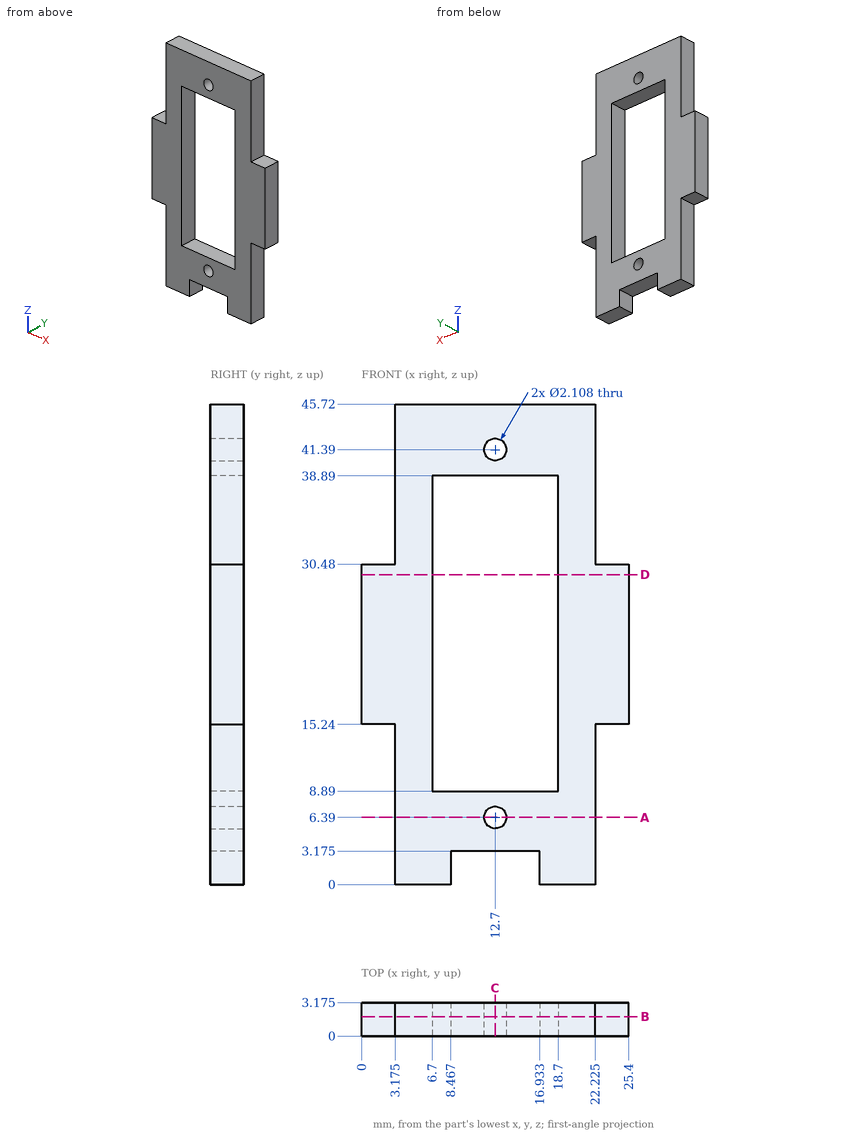
Design review of the part shown in the three views and the two pictorial views. Dimensions are in mm from the part's minimum x, y and z. Coordinates: 2 decimals unless noted, no trailing zeros. Write each loop counter-clockwise with the first axis right and the second up, starting at its lowest first coordinate (ties: lowest second). Pieces come first, ordered by that corner, then holes. Notation, with made-up numbers: (-7.5, 34.5) -> (14.5, 34.5) arc R26 ccw to (14.5, 68.5) -> close; hole circle Ø7 at (-5.5, 13). An arc over 180 degrees is marked (long way). Answer in a Markdown table with one row per item.
1. Clearance check with flat-ended pins moving along their axes: pin 1 Ø1 at (y, z) = (1, 10) entering from +X (3 decimals); pin 2 Ø1.6 at (x, y) = (13, 1) entering from -Z (3 decimals); pin 3 Ø1.6 at (y, z) = (1, 6.5) entering from -X (3 decimals); pin 4 Ø1 at (y, z) = (2, 30) entering from -X. State where each tip first meets the part, or that it passes through.
Answers below:
| item | result |
|---|---|
| pin 1 | stops at x = 22.225 |
| pin 2 | stops at z = 3.175 |
| pin 3 | stops at x = 3.175 |
| pin 4 | stops at x = 0 |
2. We need section D-D, the plane z = 29.5. State the section outline as (x, y) points (1 decimal).
Answers below:
| item | result |
|---|---|
| outline | (0, 0) -> (6.7, 0) -> (6.7, 3.2) -> (0, 3.2) -> close; (18.7, 0) -> (25.4, 0) -> (25.4, 3.2) -> (18.7, 3.2) -> close |
3. We need section C-C, the plane x = 12.7. State the section outline as (y, z) points (1 decimal).
Answers below:
| item | result |
|---|---|
| outline | (0, 3.2) -> (3.2, 3.2) -> (3.2, 5.3) -> (0, 5.3) -> close; (0, 7.4) -> (3.2, 7.4) -> (3.2, 8.9) -> (0, 8.9) -> close; (0, 38.9) -> (3.2, 38.9) -> (3.2, 40.3) -> (0, 40.3) -> close; (0, 42.4) -> (3.2, 42.4) -> (3.2, 45.7) -> (0, 45.7) -> close |
4. We need section B-B, the plane y = 1.85. State the section outline as (x, z) points (1 decimal).
Answers below:
| item | result |
|---|---|
| outline | (0, 15.2) -> (3.2, 15.2) -> (3.2, 0) -> (8.5, 0) -> (8.5, 3.2) -> (16.9, 3.2) -> (16.9, 0) -> (22.2, 0) -> (22.2, 15.2) -> (25.4, 15.2) -> (25.4, 30.5) -> (22.2, 30.5) -> (22.2, 45.7) -> (3.2, 45.7) -> (3.2, 30.5) -> (0, 30.5) -> close; hole (6.7, 8.9) -> (18.7, 8.9) -> (18.7, 38.9) -> (6.7, 38.9) -> close; hole circle Ø2.1 at (12.7, 6.4); hole circle Ø2.1 at (12.7, 41.4) |
5. Wall thickness on probe 1 along Z at (x, y) = (12.7, 1.35) (1 decimal); probe 2 along X at (y, z) = (1.1, 15.5); probe 3 along X at (y, z) = (1.6, 36) (1 decimal): over which ranges is each line inside the solid? List them lowest first. Write a range as [from, to].
Answers below:
| item | result |
|---|---|
| probe 1 | z = [3.2, 5.3], [7.4, 8.9], [38.9, 40.3], [42.4, 45.7] |
| probe 2 | x = [0, 6.7], [18.7, 25.4] |
| probe 3 | x = [3.2, 6.7], [18.7, 22.2] |
6. We need section A-A, the plane z = 6.39. State the section outline as (x, y) points (1 decimal), and give its area (3 significant figures).
Answers below:
| item | result |
|---|---|
| outline | (3.2, 0) -> (11.6, 0) -> (11.6, 3.2) -> (3.2, 3.2) -> close; (13.8, 0) -> (22.2, 0) -> (22.2, 3.2) -> (13.8, 3.2) -> close |
| area | 53.8 mm^2 |
